CAD build for the part. Positions are in the model's coordinates, mm. Face numbers are marked on the shaded views. Round coordinates to 2 decimals unless told otherwise and drop trailing zeros. Loops run counter-clockwise (first coordinate to the right, second up) from the corner with the lowest first, then second, coordinate; pieces in that order, holes last. Notation, with made-up numbers: (12, -23.75) - (68, -23.75) arc R8 cw to (68, -13.75) - close; hole circle Ø3 at (41.5, 87). An arc over 180 degrees is marked (long way). Use one line per item in the form item = value.
from build123d import *
from build123d.topology import SkipClean

# Parameters (mm, degrees)
CROQUIS1_R                 = 25.225
SALIENTE_EXTRUIR1_DEPTH    = 8
CROQUIS8_R                 = 3.5
CORTAR_EXTRUIR1_DEPTH      = 8
ROSCA1_PITCH               = 4
CORTAR_EXTRUIR2_DEPTH      = 37.559595635
CORTAR_EXTRUIR2_DEPTH_BACK = 37.559595635
CROQUIS11_W                = 9.138603142
CROQUIS11_H                = 6.021536875


with BuildPart() as part:
    # Croquis1 → Saliente-Extruir1 (new body)
    with BuildSketch(Plane.XY):
        Circle(CROQUIS1_R)
    extrude(amount=SALIENTE_EXTRUIR1_DEPTH)

    # Croquis8 → Cortar-Extruir1 (cut)
    with BuildSketch(Plane.XY.offset(8)):
        Circle(CROQUIS8_R)
    extrude(amount=-CORTAR_EXTRUIR1_DEPTH, mode=Mode.SUBTRACT)

    # Rosca1: the profile of Perfil de rosca2 profile screwed along a right-hand helix of 2 turns, 12 arcs to a turn; built about Z, then put on its axis
    with SkipClean():  # the faces are left unmerged after this step: merging them gives an invalid solid
        rosca1_z = Axis((0, 0, 0), (0, 0, 1))
        rosca1_corners = [(3.5003, 0, -0.000173205), (3.5003, 0, 3.500173194), (1.3349365, 0, 2.249999995), (1.3349365, 0, 1.249999995)]
        with BuildLine(mode=Mode.PRIVATE) as rosca1_profile:
            Line(rosca1_corners[0], rosca1_corners[1])
            Line(rosca1_corners[1], rosca1_corners[2])
            Line(rosca1_corners[2], rosca1_corners[3])
            Line(rosca1_corners[3], rosca1_corners[0])
        rosca1_cap = Face(rosca1_profile.wire())
        rosca1_turn_angles = [0, 15, 30, 45, 60, 75, 90, 105, 120, 135, 150, 165, 180, 195, 210, 225, 240, 255, 270, 285, 300, 315, 330, 345, 360]
        rosca1_turn_weights = [1, 0.9659258262890683, 1, 0.9659258262890683, 1, 0.9659258262890683, 1, 0.9659258262890683, 1, 0.9659258262890683, 1, 0.9659258262890683, 1, 0.9659258262890683, 1, 0.9659258262890683, 1, 0.9659258262890683, 1, 0.9659258262890683, 1, 0.9659258262890683, 1, 0.9659258262890683, 1]
        rosca1_turn_rails = [Edge.make_bspline([Vector(p[0], p[1], 0).rotate(rosca1_z, rosca1_turn_angles[k]) / rosca1_turn_weights[k] + Vector(0, 0, p[2] + ROSCA1_PITCH * rosca1_turn_angles[k] / 360) for k in range(25)], [0, 0, 0, 1, 1, 2, 2, 3, 3, 4, 4, 5, 5, 6, 6, 7, 7, 8, 8, 9, 9, 10, 10, 11, 11, 12, 12, 12], 2, rosca1_turn_weights) for p in rosca1_corners]
        rosca1_turn_sides = [Face.make_surface_from_curves(rosca1_turn_rails[p[0]], rosca1_turn_rails[p[1]]) for p in [(0, 1), (1, 2), (2, 3), (3, 0)]]
        rosca1 = Plane(origin=(0, 0, 8), x_dir=(-1, 0, 0), z_dir=(0, 0, -1)) * Solid(Shell([*[p.moved(Location((0, 0, ROSCA1_PITCH * i))) for i in range(2) for p in rosca1_turn_sides], rosca1_cap, rosca1_cap.rotate(rosca1_z, 720).moved(Location((0, 0, ROSCA1_PITCH * 720 / 360)))]))
        add(rosca1)

    # Croquis11 → Cortar-Extruir2 (cut, two sides: drawn at the far end of the back side and taken through both)
    with SkipClean():  # the faces are left unmerged after this step: merging them gives an invalid solid
        with BuildSketch(Plane(origin=(0, 0, 0), x_dir=(1, 0, 0), z_dir=(0, 1, 0)).offset(-CORTAR_EXTRUIR2_DEPTH_BACK)):
            with Locations((0.536755305, 3.010768438)):
                Rectangle(CROQUIS11_W, CROQUIS11_H)
        extrude(amount=CORTAR_EXTRUIR2_DEPTH + CORTAR_EXTRUIR2_DEPTH_BACK, mode=Mode.SUBTRACT)


solid = part.part
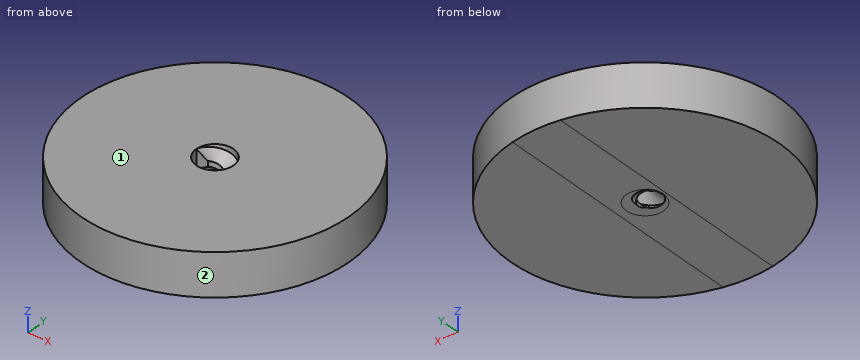
1) Two-plate mould, pull along X, no slides. Class the marked faces 1 and 2: +X half, -X half, draft (parallel to the pull), parting line (faces both ways), or undercut.
Report:
face_1 = draft
face_2 = parting line
2) Slice it at A-A (x = 16). Write the cut outline in (y, z), plus the area to 3 significant figures.
Report:
outline = (-19.5, 0) - (19.5, 0) - (19.5, 8) - (-19.5, 8) - close
area = 312 mm^2
3) Slice it at B-B (x = -14.5). Write the cut outline in (y, z), plus the area to 3 significant figures.
Report:
outline = (-20.64, 0) - (20.64, 0) - (20.64, 8) - (-20.64, 8) - close
area = 330 mm^2
4) Drill centre lines: probe 1 along X at (y, z) = (0, 4.5) (3 decimals); probe 2 along X at (y, z) = (0, 0.6) (3 decimals). Where is each one in solid material? Low to high.
Report:
probe_1 = -25.225 to -3.5, 1.335 to 25.225
probe_2 = -25.225 to -3.327, 1.335 to 25.225
5) Flat gauge pins, fed straight in: pin 1 (3 mm diameter, centred on y = 5.5, z = 1.5, fed in from -X); pin 2 (4 mm diameter, centred on x = -9.5, z = 3, fed in from +Y); pin 3 (1 mm diameter, centred on x = 13, z = 6.5, fed in from +Y). Where does each tip first touch, or does it go through?
Report:
pin_1 = -24.91
pin_2 = 24.08
pin_3 = 21.91
